Here's how the part is built. I have some questions about the finished solid (model axes, mm). A direction names the side the tool comes from. Round coordinates to 2 decimals unless told otherwise and drop trailing zeros. Order: outer loops, then holes, each group sorted by start corner. A loop starts at its lowest first (then second) coordinate and runs counter-clockwise, first axis right, second up. Notation, with made-up numbers: (64.5, 50) -> (69.5, 50) arc R17 cw to (69.5, 55) -> close; hole circle Ø8 at (-10, 69.5). An arc over 180 degrees is marked (long way). One line per item, written item: value.
Autodesk Inventor part; units mm, degrees
ref_plane "dp1_XY" through (12.7, 7.9057, 0) normal (0, 0, 1) x (1, 0, 0)
ref_plane "dp1_YZ" through (12.7, 7.9057, 0) normal (1, 0, 0) x (0, 1, 0)
ref_plane "dp1_ZX" through (12.7, 7.9057, 0) normal (0, 1, 0) x (0, 0, 1)
sketch "Sketch_2" plane through (0, 0, 0) normal (0, 0, 1) x (1, 0, 0)
  line L0 (12.7, 0) -> (0, 0)
  line L1 (0, 0) -> (0, 7.098)
  line L2 (0, 7.098) -> (0.8395, 7.9375)
  line L3 (0.8395, 7.9375) -> (6.6816, 7.9375)
  line L4 (6.6816, 7.9375) -> (7.5202, 7.0965)
  arc A0 (7.5202, 7.0965) -> (8.1407, 6.839) centre (8.1407, 7.7152) ccw
  line L5 (8.1407, 6.839) -> (9.4361, 6.839)
  arc A1 (9.4361, 6.839) -> (10.3124, 7.7153) centre (9.4361, 7.7152) ccw
  line L6 (10.3124, 7.7153) -> (10.3124, 7.9057)
  line L7 (10.3124, 7.9057) -> (12.7, 7.9057)
  line L8 (12.7, 7.9057) -> (12.7, 0)
  line L9 (12.7, 0) -> (0, 0)
revolve "Revolution1" add sketch "Sketch_2" angle 360 about axis through (12.7, 0, 0) along (1, 0, 0)
thread "Thread1"
sketch "Sketch_3" plane through (0, 0, 0) normal (0, 0, 1) x (1, 0, 0)
  line L0 (40.4876, 0) -> (12.7, 0)
  line L1 (12.7, 0) -> (12.7, 10.1918)
  line L2 (12.7, 10.1918) -> (13.462, 10.9537)
  line L3 (13.462, 10.9537) -> (34.0741, 10.9537)
  line L4 (34.0741, 10.9537) -> (34.0741, 8.9091)
  line L5 (34.0741, 8.9091) -> (34.8361, 8.9091)
  line L6 (34.8361, 8.9091) -> (35.5981, 9.671)
  line L7 (35.5981, 9.671) -> (39.7256, 9.671)
  line L8 (39.7256, 9.671) -> (40.4876, 8.9091)
  line L9 (40.4876, 8.9091) -> (40.4876, 0)
  line L10 (40.4876, 0) -> (12.7, 0)
revolve "Revolution2" add sketch "Sketch_3" angle 360 about axis through (40.4876, 0, 0) along (1, 0, 0)
sketch "Sketch3" plane through (0, 0, 0) normal (-1, 0, 0) x (0, 0, 1)
  point P0 (0, 0)
hole "Hole1" at (0, 0, 0) direction (1, 0, 0) diameter 6.4389 depth 40.4876 countersink diameter 6.9469 countersink angle 90
sketch "Sketch_10" plane through (0, 0, 0) normal (0, 0, 1) x (1, 0, 0)
  line L0 (34.0741, 0) -> (30.8991, 0)
  line L1 (30.8991, 15.3353) -> (30.8991, 10.2553)
  line L2 (30.8991, 10.2553) -> (34.0741, 10.2553)
  line L3 (34.0741, 10.2553) -> (34.0741, 15.3353)
  line L4 (34.0741, 15.3353) -> (30.8991, 15.3353)
revolve "Revolution3" cut sketch "Sketch_10" angle 360 about axis through (34.0741, 0, 0) along (1, 0, 0)
sketch "Sketch_40" plane through (0, 0, 0) normal (0, 1, 0) x (-1, 0, 0)
  line L0 (-24.6126, 10.9537) -> (-24.6126, 0)
  line L1 (-24.6126, 0) -> (-27.7876, 0)
  line L2 (-27.7876, 0) -> (-27.7876, 3.1375)
  line L3 (-27.7876, 3.1375) -> (-29.2538, 4.6037)
  line L4 (-29.2538, 4.6037) -> (-29.4521, 10.9537)
  line L5 (-29.4521, 10.9537) -> (-24.6126, 10.9537)
  line L6 (-24.6126, 10.9537) -> (-24.6126, 0)
revolve "Revolution4" cut sketch "Sketch_40" angle 360 about axis through (24.6126, 0, 10.9537) along (0, 0, 1)
thread "Thread2"
sketch "Sketch_47" plane through (0, 0, 0) normal (0, 0, 1) x (1, 0, 0)
  line L0 (34.8361, 0) -> (34.0741, 0)
  line L1 (34.0741, 9.512) -> (34.0741, 8.655)
  line L2 (34.0741, 8.655) -> (34.8361, 8.655)
  line L3 (34.8361, 8.655) -> (34.8361, 8.9091)
  line L4 (34.8361, 8.9091) -> (34.4551, 8.9091)
  line L5 (34.4551, 8.9091) -> (34.1966, 9.1676)
  arc A0 (34.1966, 9.3472) -> (34.1966, 9.1676) centre (34.2864, 9.2574) ccw
  line L6 (34.1966, 9.3472) -> (35.0205, 10.1711)
  line L7 (35.0205, 10.1711) -> (35.0205, 10.2553)
  line L8 (35.0205, 10.2553) -> (34.8173, 10.2553)
  line L9 (34.8173, 10.2553) -> (34.0741, 9.512)
revolve "Revolution5" add sketch "Sketch_47" angle 360 about axis through (34.8361, 0, 0) along (1, 0, 0)
ref_plane "dp1_XY" through (12.7, 7.9057, 0) normal (0, 0, 1) x (1, 0, 0)
ref_plane "dp1_YZ" through (12.7, 7.9057, 0) normal (1, 0, 0) x (0, 1, 0)
ref_plane "dp1_ZX" through (12.7, 7.9057, 0) normal (0, 1, 0) x (0, 0, 1)
ref_plane "dp2_XY" through (12.7, -7.9057, 0) normal (0, 0, 1) x (1, 0, 0)
ref_plane "dp2_YZ" through (12.7, -7.9057, 0) normal (1, 0, 0) x (0, 1, 0)
ref_plane "dp2_ZX" through (12.7, -7.9057, 0) normal (0, 1, 0) x (0, 0, 1)
ref_plane "hh_XY" through (0, 7.9375, 0) normal (0, 0, 1) x (1, 0, 0)
ref_plane "hh_YZ" through (0, 7.9375, 0) normal (1, 0, 0) x (0, 1, 0)
ref_plane "hh_ZX" through (0, 7.9375, 0) normal (0, 1, 0) x (0, 0, 1)
ref_plane "port_XY" through (24.6126, 0, 0) normal (0, 0, 1) x (1, 0, 0)
ref_plane "port_YZ" through (24.6126, 0, 0) normal (1, 0, 0) x (0, 1, 0)
ref_plane "port_ZX" through (24.6126, 0, 0) normal (0, 1, 0) x (0, 0, 1)
ref_plane "rod_guide_XY" through (0, 0, 0) normal (1, 0, 0) x (0, 0, -1)
ref_plane "rod_guide_YZ" through (0, 0, 0) normal (0, 0, -1) x (0, 1, 0)
ref_plane "rod_guide_ZX" through (0, 0, 0) normal (0, 1, 0) x (1, 0, 0)
ref_plane "s1_XY" through (10.3124, 0, 0) normal (0, 0, 1) x (1, 0, 0)
ref_plane "s1_YZ" through (10.3124, 0, 0) normal (1, 0, 0) x (0, 1, 0)
ref_plane "s1_ZX" through (10.3124, 0, 0) normal (0, 1, 0) x (0, 0, 1)
ref_plane "s2_XY" through (12.7, 0, 0) normal (0, 0, 1) x (1, 0, 0)
ref_plane "s2_YZ" through (12.7, 0, 0) normal (1, 0, 0) x (0, 1, 0)
ref_plane "s2_ZX" through (12.7, 0, 0) normal (0, 1, 0) x (0, 0, 1)
ref_plane "t1_XY" through (12.7, 0, 0) normal (1, 0, 0) x (0, 0, -1)
ref_plane "t1_YZ" through (12.7, 0, 0) normal (0, 0, -1) x (0, 1, 0)
ref_plane "t1_ZX" through (12.7, 0, 0) normal (0, 1, 0) x (1, 0, 0)
ref_plane "t111_XY" through (12.7, 0, 0) normal (1, 0, 0) x (0, 0, -1)
ref_plane "t111_YZ" through (12.7, 0, 0) normal (0, 0, -1) x (0, 1, 0)
ref_plane "t111_ZX" through (12.7, 0, 0) normal (0, 1, 0) x (1, 0, 0)
ref_plane "to_foot_bracket_XY" through (12.7, 0, 0) normal (1, 0, 0) x (0, 0, -1)
ref_plane "to_foot_bracket_YZ" through (12.7, 0, 0) normal (0, 0, -1) x (0, 1, 0)
ref_plane "to_foot_bracket_ZX" through (12.7, 0, 0) normal (0, 1, 0) x (1, 0, 0)
ref_plane "to_nut_XY" through (10.3124, 0, 0) normal (1, 0, 0) x (0, 0, -1)
ref_plane "to_nut_YZ" through (10.3124, 0, 0) normal (0, 0, -1) x (0, 1, 0)
ref_plane "to_nut_ZX" through (10.3124, 0, 0) normal (0, 1, 0) x (1, 0, 0)
ref_plane "to_rod_XY" through (0, 0, 0) normal (1, 0, 0) x (0, 0, -1)
ref_plane "to_rod_YZ" through (0, 0, 0) normal (0, 0, -1) x (0, 1, 0)
ref_plane "to_rod_ZX" through (0, 0, 0) normal (0, 1, 0) x (1, 0, 0)
ref_plane "to_screw_XY" through (24.6126, 2.032, -6.0452) normal (0, 1, 0) x (1, 0, 0)
ref_plane "to_screw_YZ" through (24.6126, 2.032, -6.0452) normal (1, 0, 0) x (0, 0, -1)
ref_plane "to_screw_ZX" through (24.6126, 2.032, -6.0452) normal (0, 0, -1) x (0, 1, 0)
ref_plane "to_trunnion_brackets_XY" through (11.1252, 0, 0) normal (0, 1, 0) x (1, 0, 0)
ref_plane "to_trunnion_brackets_YZ" through (11.1252, 0, 0) normal (1, 0, 0) x (0, 0, -1)
ref_plane "to_trunnion_brackets_ZX" through (11.1252, 0, 0) normal (0, 0, -1) x (0, 1, 0)
ref_plane "to_trunnion_brackets1_XY" through (11.1252, 12.7, 0) normal (0, 1, 0) x (1, 0, 0)
ref_plane "to_trunnion_brackets1_YZ" through (11.1252, 12.7, 0) normal (1, 0, 0) x (0, 0, -1)
ref_plane "to_trunnion_brackets1_ZX" through (11.1252, 12.7, 0) normal (0, 0, -1) x (0, 1, 0)
ref_plane "to_trunnion_brackets2_XY" through (11.1252, -12.7, 0) normal (0, 1, 0) x (1, 0, 0)
ref_plane "to_trunnion_brackets2_YZ" through (11.1252, -12.7, 0) normal (1, 0, 0) x (0, 0, -1)
ref_plane "to_trunnion_brackets2_ZX" through (11.1252, -12.7, 0) normal (0, 0, -1) x (0, 1, 0)
ref_plane "to_tube_XY" through (34.8361, 0, 0) normal (1, 0, 0) x (0, 0, -1)
ref_plane "to_tube_YZ" through (34.8361, 0, 0) normal (0, 0, -1) x (0, 1, 0)
ref_plane "to_tube_ZX" through (34.8361, 0, 0) normal (0, 1, 0) x (1, 0, 0)
properties part number "04R000-0_rod_guide"
Q1. For P1, Ø8, axis at y = 8.5, z = 7.5, coming from the +X side; P2, Ø10, axis at x = 4.5, z = 3, coming from the +Y side; P3, Ø1.5, axis at x = 34.5, z = 8, coming from the +Y side; P4, Ø6, axis at x = 7.5, z = 8, coming from the -Y side, each with a flat end and sliding along its axis, tell me the tip position at first contact or that it passes through.
Answers:
P1: x = 40.49
P2: y = 7.94
P3: y = 7.18
P4: y = -6.07
Q2. If we mould it in two halves opening along Z, with no side actions, what happens to faces 1 (the face through (12.7, 3, -8)), 2 (the face through (37.69, -2.1, -9.44)), 3 (the face through (34.648, -1.931, -8.697))? For each: pulls with the +Z half, pulls with the -Z half, needs draft (parallel to the pull), parting line crosses it, or undercut.
Answers:
face 1: needs draft
face 2: parting line crosses it
face 3: undercut
Q3. Which directions (+Z, -Z, +X, -X, +Y, -Y) give clear straight access to the entire face, cutting with the end or side of a thin tool? Please do faces 4 (the face through (11.52, -1.71, -7.72)), 5 (the face through (40.488, 0, -4)), 6 (the face through (24.553, -3.174, 2.143)), 7 (the face through (32.51, 9.78, 3.08)).
Answers:
face 4: none
face 5: +Z, -Z, +X, +Y, -Y
face 6: +Z
face 7: +X
Q4. I want a section at B-B on y = 0. Give the number of separate pieces and of enclosed holes in the cut face, then the cut area to 3 significant figures.
Answers:
separate pieces: 3
enclosed holes: 0
area: 448 mm2
Q5. I need wall thicknesses on line 1 along Z through (x, y) = (9.5, 0); line 2 along Z through (x, y) = (14.5, 0); line 3 along X through (y, z) = (-5.5, 6.25). Which ranges of each line are inside material? Lowest first, please.
Answers:
line 1: -6.84 to -3.22, 3.22 to 6.84
line 2: -10.95 to -3.22, 3.22 to 10.95
line 3: 12.7 to 40.49
Q6. I want a section at A-A on x = 16. Write out the boundary of the cut face in (y, z), then the cut area to 3 significant figures.
Answers:
outline: circle Ø21.91 at (0, 0); hole circle Ø6.44 at (0, 0)
area: 344 mm2
